Work out the finished part from the listing and answer in its coordinate system (mm). Face numbers are marked on the shaded views. A direction names the side the tool comes from. Coordinates: 2 decimals unless noted, no trailing zeros. Order: outer loops, then holes, each group sorted by start corner. A loop starts at its lowest first (then second) coordinate and runs counter-clockwise, first axis right, second up. Notation, with made-up numbers: M 43,3 L 47,3 A27 cw 47,36 Z; hole C 12.25,28 d9. An arc over 180 degrees is marked long. Use a Markdown table: item, result.
from build123d import *

# Parameters (mm, degrees)
F1_DEPTH = 55
F2_W     = 100
F2_H     = 29.0322554066
F3_DEPTH = 25
F4_W     = 5.3750351071
F4_H     = 18.072870967
F5_DEPTH = 29.0322554066


with BuildPart() as f1:
    # F0 (on Front) → F1 (new body)
    with BuildSketch(Plane.XZ):
        Polygon((-76.8667086959, -30.5658673523), (66.6892379522, -30.5658673523), (66.6892379522, -13.3914127946), (42.04903543, 8.0348476768), (-76.8667086959, 8.0348476768), align=None)
    extrude(amount=F1_DEPTH)

    # F2 (on face) → F3 (cut)
    with BuildSketch(Plane(origin=(0, 0, -30.5658673523), x_dir=(1, 0, 0), z_dir=(0, 0, -1))):
        with Locations((-3.8809403777, 27.016880922)):
            Rectangle(F2_W, F2_H)
    extrude(amount=-F3_DEPTH, mode=Mode.SUBTRACT)

    # F4 (on face) → F5 (join, through all)
    with BuildSketch(Plane(origin=(0, -41.5330086253, 0), x_dir=(-1, 0, 0), z_dir=(0, 1, 0))):
        with Locations((34.9972322583, -14.6023028358)):
            Rectangle(F4_W, F4_H)
    extrude(amount=F5_DEPTH)


solid = f1.part
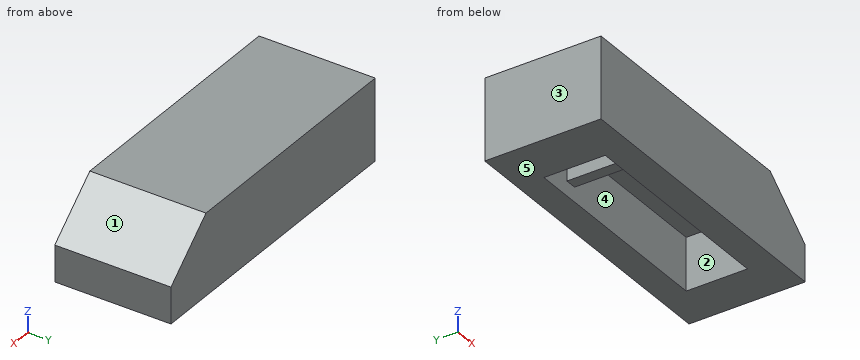
(1) A cutting plane is placed at A-A (x = 0.5). Determine the outline of the cut face in (y, z), then the cut area to 3 significant figures.
Conclusion:
| item | result |
|---|---|
| outline | M -55,-30.57 L -41.53,-30.57 L -41.53,-5.57 L -12.5,-5.57 L -12.5,-30.57 L 0,-30.57 L 0,8.03 L -55,8.03 Z |
| area | 1,400 mm2 |
(2) Straight lines are drawn through the part: L1, parallel to X at y = -41.5, z = -20.5; L2, parallel to Y at x = 11, z = -23; L3, parallel to X at y = -18, z = -11.5. For each, find the intervals that lie inside material, in ascending order.
Conclusion:
| item | result |
|---|---|
| L1 | -76.87 to -53.88, -37.68 to -32.31, 46.12 to 66.69 |
| L2 | -55 to -41.53, -12.5 to 0 |
| L3 | -76.87 to -53.88, -37.68 to -32.31, 46.12 to 64.51 |
(3) A cutting plane is placed at C-C (z = 3). Determine the outline of the cut face in (x, y), then the cut area to 3 significant figures.
Conclusion:
| item | result |
|---|---|
| outline | M -76.87,-55 L 47.84,-55 L 47.84,0 L -76.87,0 Z |
| area | 6,860 mm2 |
(4) Which of the six approach directions +Z, -Z, +X, -X, +Y, -Y give full straight-line access (tool end or side, diameter ignored) to the marked faces 4 and 5?
Conclusion:
| item | result |
|---|---|
| face 4 | -Z |
| face 5 | -Z, +X, -X, +Y, -Y |
(5) Determine the mould class of the marked faces 1, 2 and 3 for opening direction X: pulls with the +X half, pulls with the -X half, needs draft (parallel to the pull), parting line crosses it, or undercut.
Conclusion:
| item | result |
|---|---|
| face 1 | pulls with the +X half |
| face 2 | undercut |
| face 3 | pulls with the -X half |
(6) A cutting plane is placed at D-D (y = -51). Determine the outline of the cut face in (x, z), then the cut area to 3 significant figures.
Conclusion:
| item | result |
|---|---|
| outline | M -76.87,-30.57 L 66.69,-30.57 L 66.69,-13.39 L 42.05,8.03 L -76.87,8.03 Z |
| area | 5,280 mm2 |
(7) A cutting plane is placed at B-B (y = -37.5). Determine the outline of the cut face in (x, z).
Conclusion:
| item | result |
|---|---|
| outline | M -76.87,-30.57 L -53.88,-30.57 L -53.88,-5.57 L -37.68,-5.57 L -37.68,-23.64 L -32.31,-23.64 L -32.31,-5.57 L 46.12,-5.57 L 46.12,-30.57 L 66.69,-30.57 L 66.69,-13.39 L 42.05,8.03 L -76.87,8.03 Z |
(8) Given P1, Ø2, axis at y = -31, z = -1, coming from the +X side; P2, Ø1.6, axis at x = -36, y = -26.5, coming from the -Z side, each flat-ended and moving along its own axis, determine where each tip first touches the part or whether it passes through.
Conclusion:
| item | result |
|---|---|
| P1 | x = 53.59 |
| P2 | z = -23.64 |
